For this review, use the dimensioned drawing (mm, ordinates from the lowest corner) and the shaded views. A direction names the side the tool comes from. Coordinates: 2 decimals unless noted, no trailing zeros. Order: outer loops, then holes, each group sorted by start corner. A loop starts at its lowest first (then second) coordinate and runs counter-clockwise, first axis right, second up. Notation, with made-up numbers: M 2,87 L 43,87 A20 ccw 43,102 Z; hole C 81.5,32.25 d5. An arc over 180 degrees is marked long. Answer in a Markdown table with one row per item.
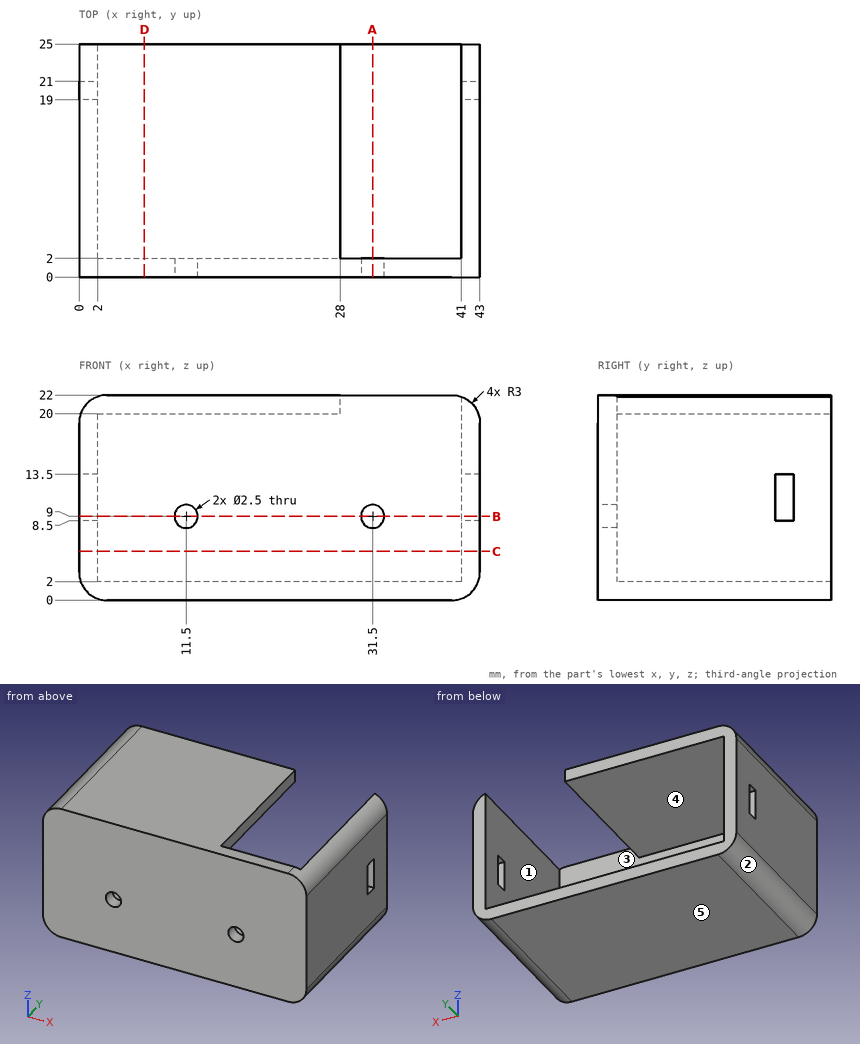
(1) To check wall thickness, follow line 1 (X direction, y = 2.75, z = 4); line 2 (Z direction, x = 11.5, y = 1.1); line 3 (Z direction, x = 11, y = 18). State the ranges of each line that lie inside material, in increasing order. Write a range as [from, to].
Report:
| item | result |
|---|---|
| line 1 | [0, 2], [41, 43] |
| line 2 | [0, 7.75], [10.25, 22] |
| line 3 | [0, 2], [20, 22] |
(2) Take a section at A-A (x = 31.5). Write out the cut boundary in (y, z).
Report:
| item | result |
|---|---|
| outline | M 0,0 L 25,0 L 25,2 L 2,2 L 2,7.75 L 0,7.75 Z; M 0,10.25 L 2,10.25 L 2,22 L 0,22 Z |
(3) Machinability: for the marked faces 4 and 5, which of the approach directions +Z, -Z, +X, -X, +Y, -Y give a long, thin tool a straight path to every point of the face, cutting with its end or side? Answer none if there is none.
Report:
| item | result |
|---|---|
| face 4 | +Y |
| face 5 | -Z, +X, -X, +Y, -Y |
(4) Take a section at D-D (x = 7). Write out the cut boundary in (y, z), then the cut area to 3 significant figures.
Report:
| item | result |
|---|---|
| outline | M 0,0 L 25,0 L 25,2 L 2,2 L 2,20 L 25,20 L 25,22 L 0,22 Z |
| area | 136 mm^2 |
(5) The part is to be moulded in two halves that separate along Z. For the marked faces 1, 2 and 3, say which applies: +Z half, -Z half, draft (parallel to the pull), parting line (faces both ways), or undercut.
Report:
| item | result |
|---|---|
| face 1 | draft |
| face 2 | -Z half |
| face 3 | undercut |
(6) Take a section at C-C (z = 5.25). Write out the cut boundary in (x, y), then the cut area to 3 significant figures.
Report:
| item | result |
|---|---|
| outline | M 0,0 L 43,0 L 43,25 L 41,25 L 41,2 L 2,2 L 2,25 L 0,25 Z |
| area | 178 mm^2 |
(7) Insertion check: P1, Ø1.5, axis at x = 31.5, z = 9, coming from the -Y side; P2, Ø4, axis at x = 11.5, z = 9, coming from the +Y side; P3, Ø0.6, axis at y = 16.5, z = 20.5, coming from the +X side; P4, Ø0.6, axis at x = 42, y = 20, coming from the +Z side. Each pin has a flat end and moves straight along its axis. Give the tip position at first contact, or say it passes through.
Report:
| item | result |
|---|---|
| P1 | through |
| P2 | y = 2 |
| P3 | x = 42.75 |
| P4 | z = 21.47 |
(8) Take a section at B-B (z = 9). Write out the cut boundary in (x, y).
Report:
| item | result |
|---|---|
| outline | M 0,0 L 10.25,0 L 10.25,2 L 2,2 L 2,19 L 0,19 Z; M 0,21 L 2,21 L 2,25 L 0,25 Z; M 12.75,0 L 30.25,0 L 30.25,2 L 12.75,2 Z; M 32.75,0 L 43,0 L 43,19 L 41,19 L 41,2 L 32.75,2 Z; M 41,21 L 43,21 L 43,25 L 41,25 Z |
